Geometry: final body of the model. Coordinates: model frame, mm. Round coordinates to 2 decimals unless told otherwise and drop trailing zeros. Write each loop counter-clockwise with the first axis right and the second up, starting at its lowest first coordinate (ties: lowest second). Pieces come first, ordered by that corner, then holes. Notation, with made-up numbers: (73, -26.75) -> (100, -26.75) arc R24 ccw to (100, -14.75) -> close; hole circle Ø5 at (50.5, 26). An arc over 180 degrees is marked (long way). Use one line per item in the form item = value. Start each with the question number.
1. Cut plane C-C, the plane z = -0.8. Return the cut outline in (x, y), plus the area to 3 significant figures.
2. Cut plane D-D, the plane x = 115.5. Return the cut outline in (y, z).
3. Line query: L1, parallel to Y at x = 76, z = -3.55; L2, parallel to Y at x = 0, z = -1.4; L3, parallel to Y at x = 8.5, z = -0.3. Output: solid intervals per line, ascending.
4. Pin query (flat end, axial travel): pin 1 Ø1.5 at (x, z) = (68, -0.5) entering from +Y. Return the tip coordinate at first contact, or that it passes through.
5. Cut plane A-A, the plane y = 0. Return the cut outline in (x, z).
6. Cut plane B-B, the plane x = 0. Return the cut outline in (y, z), plus the area to 3 significant figures.
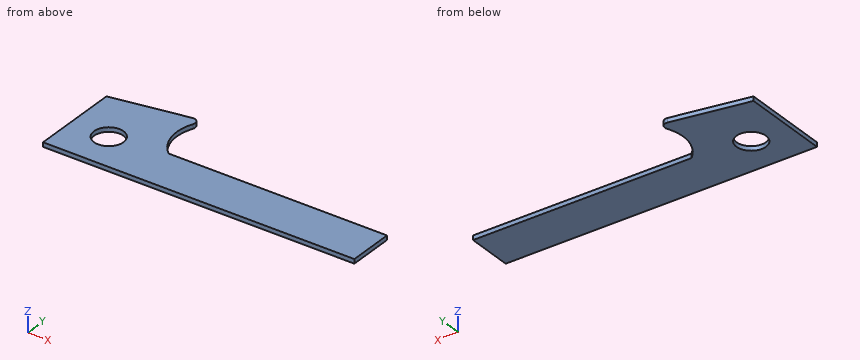
```python
from build123d import *

# Parameters (mm, degrees)
SKETCH_1_R             = 13.5
SM_BASE_FLANGE_1_DEPTH = 4


# Sheet-metal steps are written as plain solids
with BuildPart() as part:
    # Sketch 1 → Базовая кромка1 (new body)
    with BuildSketch(Plane.XY):
        with BuildLine():
            Line((0, -35), (250, -35))
            Line((250, -35), (250, 6.5))
            Line((250, 6.5), (50, 6.5))
            ThreePointArc((50, 6.5), (37.854703837, 27.206009472), (40.376084675, 51.078371856))
            ThreePointArc((40.376084675, 51.078371856), (39.763461316, 56.201257152), (34.948705483, 58.055276407))
            Line((34.948705483, 58.055276407), (-35, 45.721432364))
            Line((-35, 45.721432364), (-35, -35))
            Line((-35, -35), (0, -35))
        make_face()
        Circle(SKETCH_1_R, mode=Mode.SUBTRACT)
    extrude(amount=-SM_BASE_FLANGE_1_DEPTH)


solid = part.part
```
Outcome:
q1.outline = (-35, -35) -> (250, -35) -> (250, 6.5) -> (50, 6.5) arc R38.4 cw to (40.38, 51.08) arc R5 ccw to (34.95, 58.06) -> (-35, 45.72) -> close; hole circle Ø27 at (0, 0)
q1.area = 14,700 mm^2
q2.outline = (-35, -4) -> (6.5, -4) -> (6.5, 0) -> (-35, 0) -> close
q3.L1 = -35 to 6.5
q3.L2 = -35 to -13.5, 13.5 to 51.89
q3.L3 = -35 to -10.49, 10.49 to 53.39
q4.pin_1 = 6.5
q5.outline = (-35, -4) -> (-13.5, -4) -> (-13.5, 0) -> (-35, 0) -> close; (13.5, -4) -> (250, -4) -> (250, 0) -> (13.5, 0) -> close
q6.outline = (-35, -4) -> (-13.5, -4) -> (-13.5, 0) -> (-35, 0) -> close; (13.5, -4) -> (51.89, -4) -> (51.89, 0) -> (13.5, 0) -> close
q6.area = 240 mm^2
